Can you work these out from the model? Positions are in its coordinate system, mm. Face numbers are marked on the shaded views. A direction names the side the tool comes from. Round coordinates to 2 decimals unless told otherwise and drop trailing zeros. Loops run counter-clockwise (first coordinate to the right, second up) from the corner with the lowest first, then second, coordinate; pieces in that order, holes last. Notation, with made-up numbers: (-32.75, 13) -> (18.25, 13) arc R30 ccw to (18.25, 48) -> close; hole circle Ø5 at (44, -35.5). An arc over 180 degrees is marked (long way). Use a Markdown table: item, result.
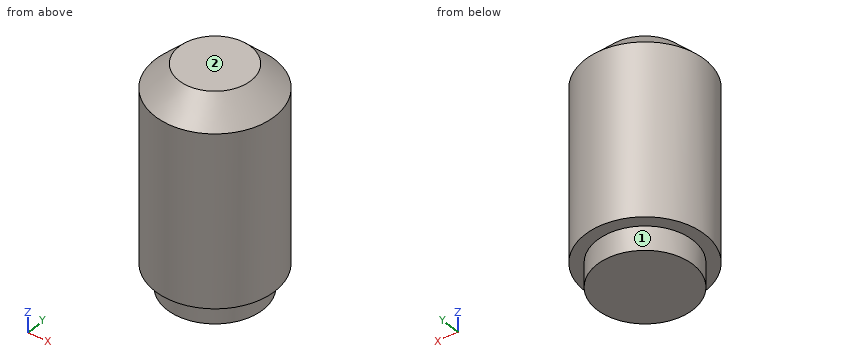
Autodesk Inventor part; units mm, degrees
ref_plane "Arbeitsebene1" through (-32.0071, -13.4173, 43.0224) normal (0, 0, 1) x (0.7071, 0.7071, 0)
ref_plane "YZ Plane" through (0, 0, 0) normal (1, 0, 0) x (0, 1, 0)
ref_plane "XZ Plane" through (0, 0, 0) normal (0, 1, 0) x (-1, 0, 0)
sketch "Skizze1" plane through (0, 0, 0) normal (0, 0, 1) x (1, 0, 0)
  circle A0 centre (-0.7274, 0.5828) radius 13
  circle A1 centre (-0.7274, 0.5828) radius 12.5
  dimension "d8" = 25
ref_plane "Arbeitsebene1" through (-32.0071, -13.4173, 43.0224) normal (0, 0, 1) x (0.7071, 0.7071, 0)
extrude "Extrusion1" add sketch "Skizze1" along normal blind 41 contours A1
chamfer "Fase1" distance 5 angle 45 1 edges at (-13.2274, 0.5828, 41)
sketch "Sketch2" plane through (-0.7274, 0.5828, 0) normal (0, 0, -1) x (-1, 0, 0)
  circle A0 centre (0, 0) radius 8.6364
  circle A1 centre (0, 0) radius 13.6364
  circle A2 centre (0, 0) radius 13.6364
  circle A3 centre (0, 0) radius 10
  point P0 (-0.7274, -0.5828)
  dimension "d5" = 20
extrude "Extrusion2" add sketch "Sketch2" along normal blind 5 contours A0 | A3
properties part number "00_Microscope_Objective_Lens10x"
1. Which directions (+Z, -Z, +X, -X, +Y, -Y) give clear straight access to the entire face, cutting with the end or side of a thin tool? Please do the marked faces 1 and 2.
Answer sheet:
| item | result |
|---|---|
| face 1 | -Z |
| face 2 | +Z, +X, -X, +Y, -Y |
2. I need wall thicknesses on line 1 (X direction, y = 0.5, z = 39.5); line 2 (Z direction, x = -5.5, y = 7); line 3 (Y direction, x = -6.5, z = 26.5). Which ranges of each line are inside material? Lowest first, please.
Answer sheet:
| item | result |
|---|---|
| line 1 | x = -9.73 to 8.27 |
| line 2 | z = -5 to 40.5 |
| line 3 | y = -10.5 to 11.67 |
3. I want a section at A-A (z = 20). Please give me the cut outline in (x, y), plus the area to 3 significant figures.
Answer sheet:
| item | result |
|---|---|
| outline | circle Ø25 at (-0.73, 0.58) |
| area | 491 mm² |
4. Will these pins go through, and if not, where does the flat tip stop? pin 1 Ø1 at (x, z) = (-8.5, 8) entering from +Y; pin 2 Ø5 at (y, z) = (8, 22.5) entering from +X.
Answer sheet:
| item | result |
|---|---|
| pin 1 | stops at y = 10.75 |
| pin 2 | stops at x = 10.76 |
